For this review, take the finished solid that the model builds, in its own axes (mm). Face numbers are marked on the shaded views. Give positions to 0.01 mm unless a question says otherwise; leave off trailing zeros. Write each loop counter-clockwise with the first axis right and the second up, starting at its lowest first coordinate (ties: lowest second). Pieces come first, ordered by that corner, then holes. Notation, with made-up numbers: (-1, 9) -> (49, 9) arc R19 ccw to (49, 15) -> close; hole circle Ø8 at (61.5, 43.25). An arc over 180 degrees is marked (long way). Return JSON: item names as keys, results as strings.
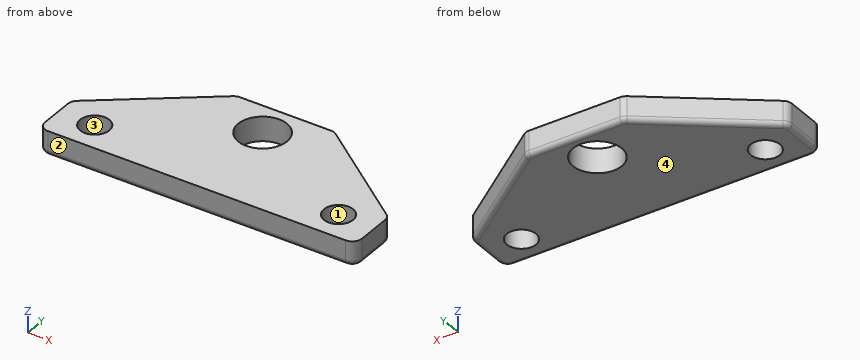
from build123d import *

# Parameters (mm, degrees)
F0_R     = 3
F0_R_2   = 5
F1_DEPTH = 5
F2_R     = 2
F3_R     = 1


with BuildPart() as f1:
    # F0 (on Top) → F1 (new body)
    with BuildSketch(Plane.XY):
        Polygon((-32.5, -24.019127), (-32.5, -34.019127), (32.5, -34.019127), (32.5, -24.019127), (10, -7.019127), (-10, -7.019127), align=None)
        with Locations((-25, -28.019127)):
            Circle(F0_R, mode=Mode.SUBTRACT)
        with Locations((25, -28.019127)):
            Circle(F0_R, mode=Mode.SUBTRACT)
        with Locations((0, -14.019127)):
            Circle(F0_R_2, mode=Mode.SUBTRACT)
    extrude(amount=F1_DEPTH)

    # F2
    f2_edges = [f1.edges().sort_by_distance(p)[0] for p in [
        (-10, -7.019127, 2.5),
        (-32.5, -24.019127, 2.5),
        (10, -7.019127, 2.5),
        (32.5, -24.019127, 2.5),
        (-32.5, -34.019127, 2.5),
        (32.5, -34.019127, 2.5),
    ]]
    fillet(f2_edges, radius=F2_R)

    # F3
    f3_edges = [f1.edges().sort_by_distance(p)[0] for p in [
        (-21.120362, -15.421178, 0),
        (-32.5, -28.516913, 0),
        (0, -34.019127, 0),
        (32.5, -28.516913, 0),
        (21.120362, -15.421178, 0),
        (0, -7.019127, 0),
    ]]
    fillet(f3_edges, radius=F3_R)


solid = f1.part
1. The part is to be moulded in two halves that separate along Y. For the marked faces 1, 2, 3 and 4, say which applies: +Y half, -Y half, draft (parallel to the pull), parting line (faces both ways), or undercut.
Results found:
{"face 1": "undercut", "face 2": "-Y half", "face 3": "undercut", "face 4": "draft"}
2. To check wall thickness, follow probe 1 along X at (y, z) = (-27.75, 1.2); probe 2 along X at (y, z) = (-30, 2.55); probe 3 along Y at (x, z) = (0, 2.4). State the ranges of each line that lie inside material, in increasing order.
Results found:
{"probe 1": "x = -32.5 to -27.99, -22.01 to 22.01, 27.99 to 32.5", "probe 2": "x = -32.5 to -27.25, -22.75 to 22.75, 27.25 to 32.5", "probe 3": "y = -34.02 to -19.02, -9.02 to -7.02"}
3. Add section C-C, the plane z = 3.9. State the section outline as (x, y) points, plus the area to 3 significant figures.
Results found:
{"outline": "(-32.5, -32.02) arc R2 ccw to (-30.5, -34.02) -> (30.5, -34.02) arc R2 ccw to (32.5, -32.02) -> (32.5, -25.01) arc R2 ccw to (31.71, -23.42) -> (10.54, -7.42) arc R2 ccw to (9.33, -7.02) -> (-9.33, -7.02) arc R2 ccw to (-10.54, -7.42) -> (-31.71, -23.42) arc R2 ccw to (-32.5, -25.01) -> close; hole circle Ø6 at (-25, -28.02); hole circle Ø10 at (0, -14.02); hole circle Ø6 at (25, -28.02)", "area": "1,240 mm²"}
4. For pin 1 (1 mm diameter, centred on y = -12.5, z = 4.5, fed in from +X), flat-tipped, find the tip position at first contact; note if it passes through.
Results found:
{"pin 1": "stops at x = 17.92"}
5. Add section A-A, the plane x = 0. State the section outline as (y, z) points, plus the area to 3 significant figures.
Results found:
{"outline": "(-34.02, 1) arc R1 ccw to (-33.02, 0) -> (-19.02, 0) -> (-19.02, 5) -> (-34.02, 5) -> close; (-9.02, 0) -> (-8.02, 0) arc R1 ccw to (-7.02, 1) -> (-7.02, 5) -> (-9.02, 5) -> close", "area": "84.6 mm²"}
6. Add section B-B, the plane y = -26.25. State the section outline as (x, z) points, plus the area to 3 significant figures.
Results found:
{"outline": "(-32.5, 1) arc R1 ccw to (-31.5, 0) -> (-27.42, 0) -> (-27.42, 5) -> (-32.5, 5) -> close; (-22.58, 0) -> (22.58, 0) -> (22.58, 5) -> (-22.58, 5) -> close; (27.42, 0) -> (31.5, 0) arc R1 ccw to (32.5, 1) -> (32.5, 5) -> (27.42, 5) -> close", "area": "276 mm²"}
